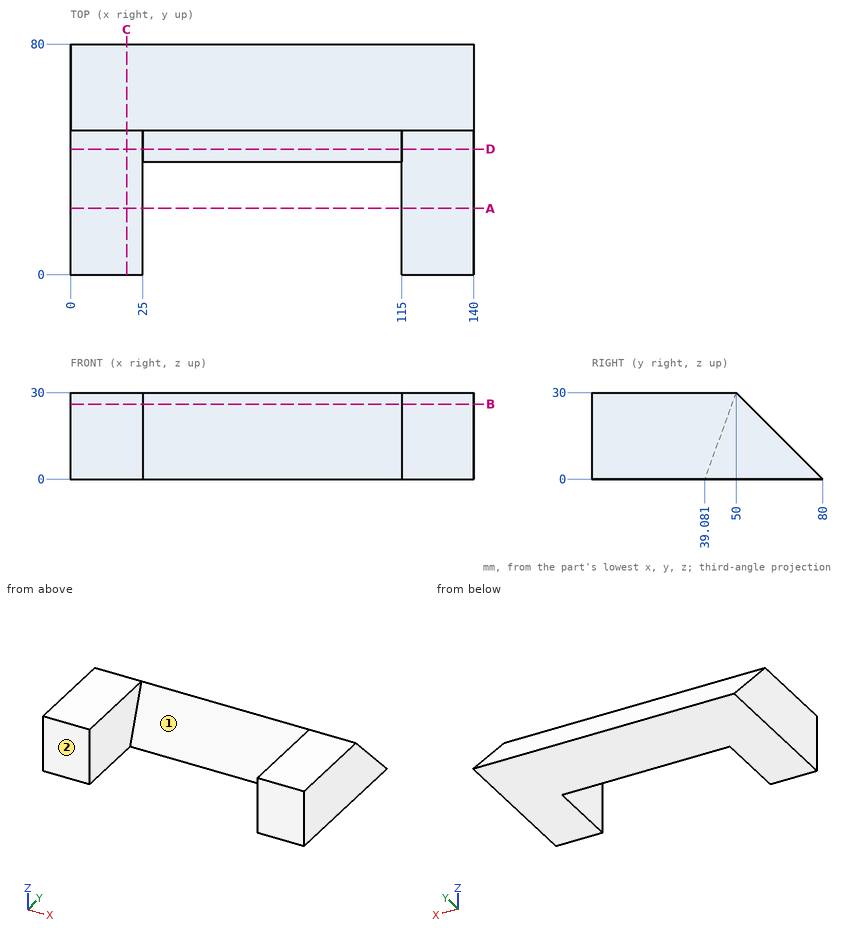
Can you work these out from the drawing? Everything is in mm from the part's minimum corner. A direction names the side the tool comes from. Round coordinates to 2 decimals unless told otherwise and drop trailing zeros. Loops run counter-clockwise (first coordinate to the right, second up) from the corner with the lowest first, then second, coordinate; pieces in that order, holes last. Notation, with made-up numbers: (64, 85.5) -> (91, 85.5) arc R15 cw to (91, 99.5) -> close; hole circle Ø3 at (-23, 9.5). An arc over 180 degrees is marked (long way). Put each result on its own line as item: value.
Q1. I want a section at B-B on z = 26. Write out the boundary of the cut face in (x, y).
Checks:
outline: (0, 0) -> (25, 0) -> (25, 48.54) -> (115, 48.54) -> (115, 0) -> (140, 0) -> (140, 54) -> (0, 54) -> close
Q2. Which directions (+Z, -Z, +X, -X, +Y, -Y) give clear straight access to the entire face, cutting with the end or side of a thin tool? Please do the marked faces 1 and 2.
Checks:
face 1: +Z, -Y
face 2: +Z, -Z, +X, -X, -Y
Q3. I want a section at D-D on y = 43.5. Write out the boundary of the cut face in (x, z).
Checks:
outline: (0, 0) -> (140, 0) -> (140, 30) -> (115, 30) -> (115, 12.14) -> (25, 12.14) -> (25, 30) -> (0, 30) -> close
Q4. I want a section at A-A on y = 23. Write out the boundary of the cut face in (x, z).
Checks:
outline: (0, 0) -> (25, 0) -> (25, 30) -> (0, 30) -> close; (115, 0) -> (140, 0) -> (140, 30) -> (115, 30) -> close
Q5. Please list where these lines run through material, in increasing order: line 1 (X direction, y = 18, z = 19.5); line 2 (Z direction, x = 75.5, y = 75); line 3 (Y direction, x = 107, z = 8). Write a range as from..to.
Checks:
line 1: 0..25, 115..140
line 2: 0..5
line 3: 41.99..72
Q6. I want a section at C-C on x = 19.5. Write out the boundary of the cut face in (y, z), and give its area (3 significant figures).
Checks:
outline: (0, 0) -> (80, 0) -> (50, 30) -> (0, 30) -> close
area: 1,950 mm2
Q7. For pin 1 Ø6 at (x, z) = (74.5, 15) entering from -Y; pin 2 Ø3 at (x, y) = (47.5, 44) entering from -Z; pin 3 Ø2 at (x, z) = (66, 22) entering from -Y, each with a flat end and sliding along its axis, tell me the tip position at first contact or that it passes through.
Checks:
pin 1: y = 43.45
pin 2: z = 0
pin 3: y = 46.72
